The drawing under review shows one solid part. Ordinate dimensions are in mm from its lowest x, y, z. Round coordinates to 2 decimals unless told otherwise and drop trailing zeros. Order: outer loops, then holes, each group sorted by start corner. A loop starts at its lowest first (then second) coordinate and runs counter-clockwise, first axis right, second up.
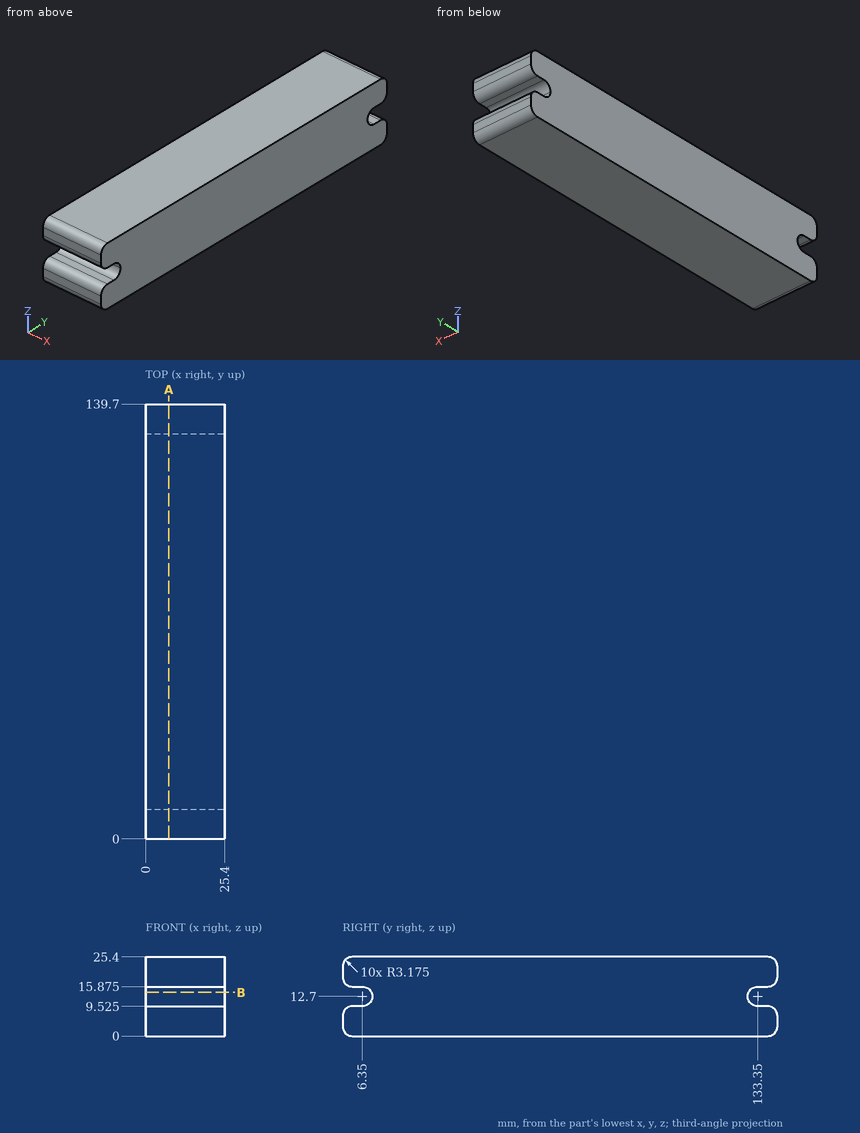
Q1. Wall thickness on line 1 (Y direction, x = 22.5, z = 18); line 2 (Y direction, x = 16, z = 12.25); line 3 (Z direction, x = 4, y = 8): over which ranges is each line inside the solid? List them lowest first.
Q2. Clearance check with flat-ended pins moving along their axes: pin 1 (5 mm diameter, centred on y = 69.5, z = 15, fed in from -X); pin 2 (2 mm diameter, centred on x = 12, z = 12.5, fed in from +Y); pin 3 (8 mm diameter, centred on x = 11.5, z = 11.5, fed in from -Y). State where each tip first meets the part, or that it passes through.
Q3. Take a section at A-A, the plane x = 7.5. State the section outline as (y, z) points (3 decimals).
Q4. Take a section at B-B, the plane z = 14. State the section outline as (x, y) points.
Working result:
1. line 1: y = 0.18 to 139.52
1. line 2: y = 9.49 to 130.21
1. line 3: z = 0 to 9.99, 15.41 to 25.4
2. pin 1: stops at x = 0
2. pin 2: stops at y = 130.41
2. pin 3: stops at y = 0.22
3. outline: (0, 3.175) arc R3.175 ccw to (3.175, 0) - (136.525, 0) arc R3.175 ccw to (139.7, 3.175) - (139.7, 6.35) arc R3.175 ccw to (136.525, 9.525) - (133.35, 9.525) arc R3.175 cw to (133.35, 15.875) - (136.525, 15.875) arc R3.175 ccw to (139.7, 19.05) - (139.7, 22.225) arc R3.175 ccw to (136.525, 25.4) - (3.175, 25.4) arc R3.175 ccw to (0, 22.225) - (0, 19.05) arc R3.175 ccw to (3.175, 15.875) - (6.35, 15.875) arc R3.175 cw to (6.35, 9.525) - (3.175, 9.525) arc R3.175 ccw to (0, 6.35) - close
4. outline: (0, 9.25) - (25.4, 9.25) - (25.4, 130.45) - (0, 130.45) - close
